from build123d import *

# Parameters (mm, degrees)
SKETCH1_R           = 1.7859375
BOSS_EXTRUDE1_DEPTH = 1.5875
FILLET1_R           = 3.175


with BuildPart() as part:
    # Sketch1 → Boss-Extrude1 (new body)
    with BuildSketch(Plane.XY):
        with BuildLine():
            ThreePointArc((33.144558463, -2.205331856), (29.617756121, 8.980256121), (18.432168144, 12.507058463))
            Line((18.432168144, 12.507058463), (12.178638912, 11.404392535))
            ThreePointArc((12.178638912, 11.404392535), (9.43473159, 9.087090354), (10.092061938, 5.55625))
            Line((10.092061938, 5.55625), (-10.092061938, 5.55625))
            ThreePointArc((-10.092061938, 5.55625), (-9.43473159, 9.087090354), (-12.178638912, 11.404392535))
            Line((-12.178638912, 11.404392535), (-18.432168144, 12.507058463))
            ThreePointArc((-18.432168144, 12.507058463), (-29.617756121, 8.980256121), (-33.144558463, -2.205331856))
            ThreePointArc((-33.144558463, -2.205331856), (-29.006698655, -5.102692459), (-26.109338088, -0.964832626))
            ThreePointArc((-26.109338088, -0.964832626), (-20.153240935, -5.535106794), (-15.08125, 0))
            Line((-15.08125, 0), (7.9375, 0))
            ThreePointArc((7.9375, 0), (8.370242006, -3.287001873), (9.638977372, -6.35))
            ThreePointArc((9.638977372, -6.35), (14.51824938, -7.657396978), (15.825646329, -2.778124963))
            ThreePointArc((15.825646329, -2.778124963), (21.602332634, -5.471838087), (26.109338066, -0.964832752))
            ThreePointArc((26.109338066, -0.964832752), (29.006698718, -5.10269247), (33.144558463, -2.205331856))
        make_face()
        with Locations((-20.6375, 0)):
            Circle(SKETCH1_R, mode=Mode.SUBTRACT)
        with Locations((12.732311861, -4.5640625)):
            Circle(SKETCH1_R, mode=Mode.SUBTRACT)
        with Locations((20.6375, 0)):
            Circle(SKETCH1_R, mode=Mode.SUBTRACT)
        with BuildLine():
            ThreePointArc((-31.385753367, -1.895207064), (-28.354907604, 7.717407604), (-18.742292936, 10.748253367))
            ThreePointArc((-18.742292936, 10.748253367), (-17.293612632, 8.679323478), (-19.362542521, 7.230643174))
            ThreePointArc((-19.362542521, 7.230643174), (-25.82921057, 5.19171057), (-27.868143174, -1.274957479))
            ThreePointArc((-27.868143174, -1.274957479), (-29.316823478, -3.343887368), (-31.385753367, -1.895207064))
        make_face(mode=Mode.SUBTRACT)
        with Locations((-12.798888497, 7.886782342)):
            Circle(SKETCH1_R, mode=Mode.SUBTRACT)
        with BuildLine():
            ThreePointArc((18.742292936, 10.748253367), (28.354907604, 7.717407604), (31.385753367, -1.895207064))
            ThreePointArc((31.385753367, -1.895207064), (29.316823478, -3.343887368), (27.868143174, -1.274957479))
            ThreePointArc((27.868143174, -1.274957479), (25.82921057, 5.19171057), (19.362542521, 7.230643174))
            ThreePointArc((19.362542521, 7.230643174), (17.293612632, 8.679323478), (18.742292936, 10.748253367))
        make_face(mode=Mode.SUBTRACT)
        with Locations((12.798888497, 7.886782342)):
            Circle(SKETCH1_R, mode=Mode.SUBTRACT)
    extrude(amount=BOSS_EXTRUDE1_DEPTH)

    # Fillet1
    fillet1_edges = [part.edges().sort_by_distance(p)[0] for p in [
        (26.109338066, -0.964832752, 0.79375),
        (15.825646329, -2.778124963, 0.79375),
        (7.9375, 0, 0.79375),
        (-15.08125, 0, 0.79375),
        (-26.109338088, -0.964832626, 0.79375),
        (-10.092061938, 5.55625, 0.79375),
        (10.092061938, 5.55625, 0.79375),
    ]]
    fillet(fillet1_edges, radius=FILLET1_R)


solid = part.part
Check sheet for the modelled part. Datum: model origin and axes. Units: mm. A direction names the side the tool comes from. Round coordinates to 2 decimals unless told otherwise and drop trailing zeros. Order: outer loops, then holes, each group sorted by start corner. A loop starts at its lowest first (then second) coordinate and runs counter-clockwise, first axis right, second up. Notation, with made-up numbers: M -23.5,9.25 L -6.5,9.25 A35 cw -6.5,48.25 Z; hole C 46.25,45 d7. An arc over 180 degrees is marked long. One line per item, written item: value. Start each with the question number.
1. Section check B-B on y = 4.5. Enter the section's corners in (x, z).
2. Release check for a two-part mould opening along Y. For faces 1 (the cylindrical face through (25.9, 5.12, 0.78)), 2 (the flat face through (0, 5.556, 1)), 3 (the flat face through (0, 2, 0)), 4 (the cylindrical face through (-31.03, -4.87, 0.78)) record: released by +Y, released by -Y, zero draft, split by the parting line, or undercut.
3. Gauge pin test, flat ends, axial feed: P1, Ø0.5, axis at x = -6.5, z = 1, coming from the -Y side; P2, Ø3, axis at x = 20.64, y = 0, coming from the -Z side. Record the tip position at first contact, or that the pin passes through.
4. Section check C-C on z = 0.35. Give the number of separate pieces and of enclosed holes in the cut face, and give its area (3 significant figures).
5. Scan lines: line 1 along X through (y, z) = (1.25, 0.5); line 2 along X through (y, z) = (-1, 1.2); line 3 along X through (y, z) = (-0.5, 0.2). Record each from-to range of solid material in increasing order.
6. Access from +Z, -Z, +X, -X, +Y, -Y to the whole of each face (thin tool, end or side, straight path). Record for faces 5 (the cylindrical face through (8.753, -4.477, 0.783)), 6 (the flat face through (15.349, 11.963, 0.783)), 7 (the flat face through (0, 2, 1.588)).
7. Section check A-A on x = 13.5. Enter the section's corners in (y, z).
Results found:
1. outline: M -32.51,0 L -30.58,0 L -30.58,1.59 L -32.51,1.59 Z; M -26.44,0 L 26.44,0 L 26.44,1.59 L -26.44,1.59 Z; M 30.58,0 L 32.51,0 L 32.51,1.59 L 30.58,1.59 Z
2. face 1: undercut
2. face 2: released by +Y
2. face 3: zero draft
2. face 4: released by -Y
3. P1: y = 0
3. P2: through
4. separate pieces: 1
4. enclosed holes: 7
4. area: 656 mm^2
5. line 1: -33.28 to -31.48, -27.87 to -21.91, -19.36 to 19.36, 21.91 to 27.87, 31.48 to 33.28
5. line 2: -33.3 to -31.51, -27.91 to -22.12, -19.16 to -14.82, 7.4 to 19.16, 22.12 to 27.91, 31.51 to 33.3
5. line 3: -33.33 to -31.54, -27.96 to -22.35, -18.92 to -14.21, 6.79 to 18.92, 22.35 to 27.96, 31.54 to 33.33
6. face 5: +Z, -Z, -Y
6. face 6: +Z, -Z, +Y
6. face 7: +Z, +X, -X, +Y, -Y
7. outline: M -8.05,0 L -6.18,0 L -6.18,1.59 L -8.05,1.59 Z; M -2.95,0 L 6.24,0 L 6.24,1.59 L -2.95,1.59 Z; M 9.53,0 L 11.64,0 L 11.64,1.59 L 9.53,1.59 Z
